Part model, mm, in its own coordinate system. Face numbers are marked on the shaded views. Give positions to 0.01 mm unless a question says otherwise; leave off trailing zeros. Order: outer loops, then holes, each group sorted by start corner. A loop starts at its lowest first (then second) coordinate and runs counter-clockwise, first axis right, second up.
1. Slice it at C-C on x = -8.75. List the corners of the cut face in (y, z), and give its area (3 significant figures).
2. Slice it at A-A on y = -3.5. Give the number of separate pieces and of enclosed holes in the cut face, and give its area (3 significant figures).
3. Drop flat-ended pins along their axis: pin 1 Ø3 at (x, z) = (5.5, 1) entering from -Y; pin 2 Ø4 at (x, y) = (-4.5, -6) entering from +Z; pin 3 Ø4 at (y, z) = (-4.5, -0.5) entering from +X; pin 4 Ø0.7 at (y, z) = (-5.5, -1) entering from +X. Give the stop position or say it passes through.
4. Probe line 1 (Z direction, x = 4, y = -0.5); line 2 (Y direction, x = 1, z = -1.5); line 3 (Y direction, x = 1, z = 1.5). List the from-to ranges inside material, lowest first.
5. Mould opens along X. For the marked faces 1, 2, 3 and 4 say: +X half, -X half, draft (parallel to the pull), parting line (faces both ways), or undercut.
from build123d import *

# Parameters (mm, degrees)
CROQUIS1_W              = 20
CROQUIS1_H              = 2.5
SALIENTE_EXTRUIR1_DEPTH = 3
CROQUIS2_R              = 0.461571169
SALIENTE_EXTRUIR2_DEPTH = 3
MATRIZL1_COUNT          = 8
MATRIZL1_PITCH          = 2.5
SALIENTE_EXTRUIR3_DEPTH = 0.45
MATRIZL2_COUNT          = 8
MATRIZL2_PITCH          = 2.5


with BuildPart() as part:
    # Croquis1 → Saliente-Extruir1 (new body)
    with BuildSketch(Plane.XY):
        Rectangle(CROQUIS1_W, CROQUIS1_H)
    extrude(amount=SALIENTE_EXTRUIR1_DEPTH)

    # Croquis2 → Saliente-Extruir2 (add)
    with BuildSketch(Plane.XY.offset(3)):
        with Locations((-8.75, 0)):
            Circle(CROQUIS2_R)
    saliente_extruir2 = extrude(amount=SALIENTE_EXTRUIR2_DEPTH)

    # MatrizL1: Saliente-Extruir2 ×8
    with Locations(*[(i * MATRIZL1_PITCH, 0, 0) for i in range(1, MATRIZL1_COUNT)]):
        add(saliente_extruir2)

    # Croquis3 → Saliente-Extruir3 (add, symmetric)
    with BuildSketch(Plane(origin=(8.75, 0, 0), x_dir=(0, 0, -1), z_dir=(1, 0, 0))):
        with BuildLine():
            Line((0, -0.45), (1.55, -0.45))
            Line((1.55, -0.45), (1.55, -7))
            ThreePointArc((1.55, -7), (2, -7.45), (2.45, -7))
            Line((2.45, -7), (2.45, -0.4))
            ThreePointArc((2.45, -0.4), (2.201040764, 0.201040764), (1.6, 0.45))
            Line((1.6, 0.45), (0, 0.45))
            Line((0, 0.45), (0, -0.45))
        make_face()
    saliente_extruir3 = extrude(amount=SALIENTE_EXTRUIR3_DEPTH, both=True)

    # MatrizL2: Saliente-Extruir3 ×8
    with Locations(*[(-i * MATRIZL2_PITCH, 0, 0) for i in range(1, MATRIZL2_COUNT)]):
        add(saliente_extruir3)


solid = part.part
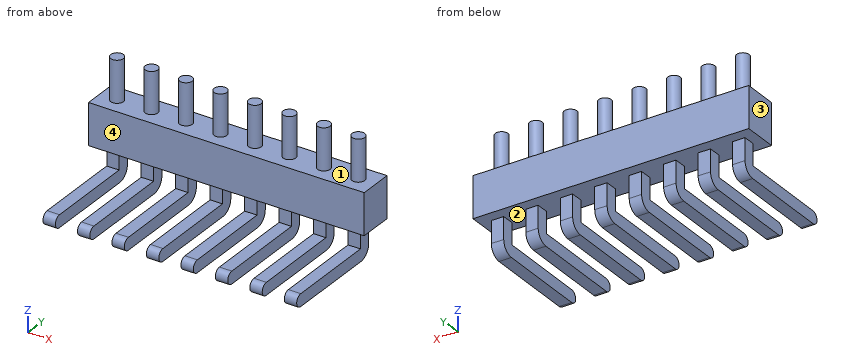
Data:
1. outline: (-7, -2.45) - (-0.4, -2.45) arc R0.85 ccw to (0.45, -1.6) - (0.45, 0) - (1.25, 0) - (1.25, 3) - (0.46, 3) - (0.46, 6) - (-0.46, 6) - (-0.46, 3) - (-1.25, 3) - (-1.25, 0) - (-0.45, 0) - (-0.45, -1.55) - (-7, -1.55) arc R0.45 ccw to start
1. area: 18.5 mm2
2. separate pieces: 8
2. enclosed holes: 0
2. area: 6.48 mm2
3. pin 1: stops at y = -1.25
3. pin 2: stops at z = -1.55
3. pin 3: stops at x = 9.2
3. pin 4: passes through
4. line 1: z = -2.45 to -1.55, 0 to 3
4. line 2: y = -0.45 to 0.45
4. line 3: y = -1.25 to 1.25
5. face 1: undercut
5. face 2: undercut
5. face 3: -X half
5. face 4: draft
